```python
from build123d import *

# Parameters (mm, degrees)
SKETCH1_R           = 10
BOSS_EXTRUDE1_DEPTH = 100
SKETCH2_R           = 10
SKETCH2_R_2         = 2.5
CUT_EXTRUDE2_DEPTH  = 20
SKETCH3_R           = 10
SKETCH3_R_2         = 2.5
CUT_EXTRUDE3_DEPTH  = 20


with BuildPart() as part:
    # Sketch1 → Boss-Extrude1 (new body)
    with BuildSketch(Plane(origin=(0, 0, 0), x_dir=(1, 0, 0), z_dir=(0, 1, 0))):
        Circle(SKETCH1_R)
    extrude(amount=BOSS_EXTRUDE1_DEPTH)

    # Sketch2 → Cut-Extrude2 (cut)
    with BuildSketch(Plane(origin=(0, 100, 0), x_dir=(1, 0, 0), z_dir=(0, 1, 0))):
        Circle(SKETCH2_R)
        Circle(SKETCH2_R_2, mode=Mode.SUBTRACT)
    extrude(amount=-CUT_EXTRUDE2_DEPTH, mode=Mode.SUBTRACT)

    # Sketch3 → Cut-Extrude3 (cut)
    with BuildSketch(Plane.XZ):
        Circle(SKETCH3_R)
        Circle(SKETCH3_R_2, mode=Mode.SUBTRACT)
    extrude(amount=-CUT_EXTRUDE3_DEPTH, mode=Mode.SUBTRACT)


solid = part.part
```
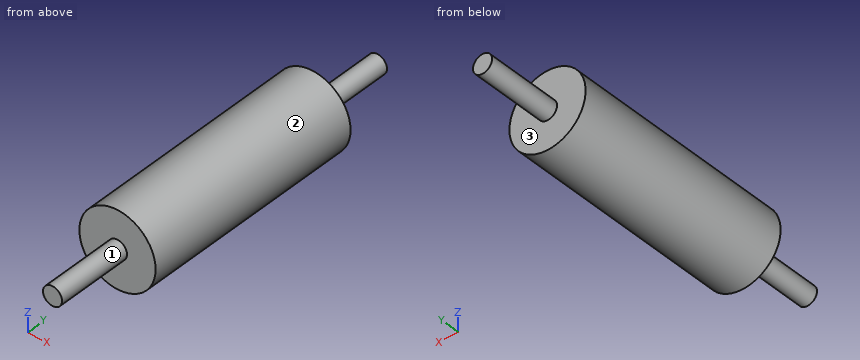
The model under review builds one solid part; all positions refer to its coordinate system, in mm. Face numbers are marked on the shaded views. A direction names the side the tool comes from. Round coordinates to 2 decimals unless told otherwise and drop trailing zeros. Loops run counter-clockwise (first coordinate to the right, second up) from the corner with the lowest first, then second, coordinate; pieces in that order, holes last. Notation, with made-up numbers: M 46.5,63.5 L 59.5,63.5 A23 ccw 59.5,95.5 Z; hole C 77,38.25 d10. An arc over 180 degrees is marked long. Answer as a JSON object with one key per item and string values.
(1) Take a section at D-D on y = 58.5. Give the boundary of the cut face in (x, z), and give its area (3 significant figures).
Resolved:
{"outline": "C 0,0 d20", "area": "314 mm²"}
(2) Take a section at C-C on y = 91. Give the boundary of the cut face in (x, z).
Resolved:
{"outline": "C 0,0 d5"}
(3) To check wall thickness, follow line 1 along Y through (x, z) = (2.25, -8.25); line 2 along Z through (x, y) = (0, 16); line 3 along X through (y, z) = (76.5, 0.5). State the ranges of each line that lie inside material, in increasing order.
Resolved:
{"line 1": "20 to 80", "line 2": "-2.5 to 2.5", "line 3": "-9.99 to 9.99"}
(4) Clearance check with flat-ended pins moving along their axes: P1, Ø1.5, axis at x = 4, z = -6.5, coming from the -Y side; P2, Ø1.5, axis at y = 42.5, z = -2, coming from the +X side; P3, Ø1, axis at y = 48.5, z = -7, coming from the +X side. State where each tip first meets the part, or that it passes through.
Resolved:
{"P1": "y = 20", "P2": "x = 9.92", "P3": "x = 7.6"}
(5) Take a section at A-A on z = 0. Give the boundary of the cut face in (x, y).
Resolved:
{"outline": "M -10,20 L -2.5,20 L -2.5,0 L 2.5,0 L 2.5,20 L 10,20 L 10,80 L 2.5,80 L 2.5,100 L -2.5,100 L -2.5,80 L -10,80 Z"}
(6) Tool access review of the marked faces 1, 2 and 3: name each direction out of +Z, -Z, +X, -X, +Y, -Y from which nothing blocks a thin tool from reaching the whole face with its end or side.
Resolved:
{"face 1": "-Y", "face 2": "+Y, -Y", "face 3": "+Y"}
(7) Take a section at B-B on x = 0. Give the boundary of the cut face in (y, z).
Resolved:
{"outline": "M 0,-2.5 L 20,-2.5 L 20,-10 L 80,-10 L 80,-2.5 L 100,-2.5 L 100,2.5 L 80,2.5 L 80,10 L 20,10 L 20,2.5 L 0,2.5 Z"}
